from build123d import *

# Parameters (mm, degrees)
SKETCH1_R           = 15.875
SKETCH1_R_2         = 6.35
BOSS_EXTRUDE1_DEPTH = 215.9
BOSS_EXTRUDE2_START = 12.7
SKETCH2_R           = 15.875
SKETCH2_R_2         = 12.7
BOSS_EXTRUDE2_DEPTH = 12.7
SKETCH3_W           = 3.81
SKETCH3_H           = 6.35
CUT_EXTRUDE1_START  = -25.4
SKETCH4_R           = 15.875
CUT_EXTRUDE1_DEPTH  = 25.4


with BuildPart() as part:
    # Sketch1 → Boss-Extrude1 (new body)
    with BuildSketch(Plane(origin=(0, 0, 0), x_dir=(1, 0, 0), z_dir=(0, 1, 0))):
        with Locations(Location((0, 0, 0), (0, 0, 270))):
            Circle(SKETCH1_R)
        with Locations(Location((0, 0, 0), (0, 0, 270))):
            Circle(SKETCH1_R_2, mode=Mode.SUBTRACT)
    extrude(amount=BOSS_EXTRUDE1_DEPTH)

    # Sketch2 → Boss-Extrude2 (add)
    with BuildSketch(Plane.XZ.offset(BOSS_EXTRUDE2_START)):
        with Locations(Location((0, 0, 0), (0, 0, 270))):
            Circle(SKETCH2_R)
        with Locations(Location((0, 0, 0), (0, 0, 270))):
            Circle(SKETCH2_R_2, mode=Mode.SUBTRACT)
    extrude(amount=-BOSS_EXTRUDE2_DEPTH)

    # Sketch3 → Cut-Revolve1 (revolve, cut)
    with BuildSketch(Plane(origin=(0, 0, 0), x_dir=(0, 0, -1), z_dir=(1, 0, 0))):
        with Locations((13.97, 174.625)):
            Rectangle(SKETCH3_W, SKETCH3_H)
    revolve(axis=Axis((0, -12.7, 0), (0, 1, 0)), mode=Mode.SUBTRACT)

    # Sketch4 → Cut-Extrude1 (cut)
    with BuildSketch(Plane(origin=(0, 215.9, 0), x_dir=(1, 0, 0), z_dir=(0, 1, 0)).offset(CUT_EXTRUDE1_START)):
        with Locations(Location((0, 0, 0), (0, 0, 90))):
            Circle(SKETCH4_R)
        Polygon((9.592403624, 11.092300304), (-4.810012038, 13.853415374), (-14.402415662, 2.76111507), (-9.592403624, -11.092300304), (4.810012038, -13.853415374), (14.402415662, -2.76111507), align=None, mode=Mode.SUBTRACT)
    extrude(amount=CUT_EXTRUDE1_DEPTH, mode=Mode.SUBTRACT)


solid = part.part
The listing builds one solid part. Answer for the finished solid, in the listing's coordinates (mm). A direction names the side the tool comes from. Give positions to 0.01 mm unless a question says otherwise; leave off trailing zeros. Order: outer loops, then holes, each group sorted by start corner. A loop starts at its lowest first (then second) coordinate and runs counter-clockwise, first axis right, second up. Notation, with made-up numbers: (-39, 69) - (4, 69) arc R27 ccw to (4, 85) - close; hole circle Ø6 at (-38, 83). An arc over 180 degrees is marked (long way). One line per item, written item: value. Start each with the question number.
1) A cutting plane is placed at C-C on y = 38.5. Give the vertices of the cut face in (x, z) (3 decimals), then the cut area to 3 significant figures.
2) A cutting plane is placed at B-B on x = 0. Give the vertices of the cut face in (y, z) (3 decimals), then the cut area to 3 significant figures.
3) Find the intervals of material crossed by L1, parallel to Y at x = -13.5, z = -7; L2, parallel to X at y = 168, z = 0 (3 decimals); L3, parallel to X at y = -8.5, z = 0 (3 decimals), in increasing order.
4) Given pin 1 Ø3 at (y, z) = (62, 7) entering from +X; pin 2 Ø1 at (x, z) = (-4.5, 9) entering from -Y; pin 3 Ø3 at (y, z) = (123, -6.5) entering from +X, each flat-ended and moving along its own axis, determine where each tip first touches the part or whether it passes through.
5) A tool of negligible diameter and unlimited length cuts with its end or side. For faces 1 (the face through (9.539, 203.022, 8.385)), 2 (the face through (-7.7, -6.4, 10.1)), 3 (the face through (-9.539, 203.022, -8.385)), 4 (the face through (-2.492, 203.022, 12.454)), 5 (the face through (12.03, 203.02, -4.07)), from which of +Z, -Z, +X, -X, +Y, -Y can it reach the whole face along a straight path? Write none if from no direction.
6) The mould has two halves that part along Y. Classify faces 6 (the face through (-12.03, 203.02, 4.07)), 7 (the face through (13, 190.5, -2)), 8 (the face through (-6, 177.8, 11)), 9 (the face through (-6, 171.45, 11)): released by +Y, released by -Y, zero draft, split by the parting line, or undercut.
7) A cutting plane is placed at D-D on z = 8.5. Give the vertices of the cut face in (x, y), then the cut area to 3 significant figures.
8) A cutting plane is placed at A-A on z = 0. Give the vertices of the cut face in (x, y) (3 decimals).
Answer sheet:
1. outline: circle Ø31.75 at (0, 0); hole circle Ø12.7 at (0, 0)
1. area: 665 mm2
2. outline: (-12.7, -15.875) - (171.45, -15.875) - (171.45, -12.065) - (177.8, -12.065) - (177.8, -15.875) - (190.5, -15.875) - (190.5, -12.931) - (215.9, -12.931) - (215.9, -6.35) - (0, -6.35) - (0, -12.7) - (-12.7, -12.7) - close; (-12.7, 12.7) - (0, 12.7) - (0, 6.35) - (215.9, 6.35) - (215.9, 12.931) - (190.5, 12.931) - (190.5, 15.875) - (177.8, 15.875) - (177.8, 12.065) - (171.45, 12.065) - (171.45, 15.875) - (-12.7, 15.875) - close
2. area: 4,000 mm2
3. L1: y = -12.7 to 171.45, 177.8 to 190.5
3. L2: x = -15.875 to -6.35, 6.35 to 15.875
3. L3: x = -15.875 to -12.7, 12.7 to 15.875
4. pin 1: stops at x = 14.89
4. pin 2: stops at y = 0
4. pin 3: stops at x = 15.07
5. face 1: +Z, +X, +Y
5. face 2: -Y
5. face 3: -Z, -X, +Y
5. face 4: +Z, -X, +Y
5. face 5: -Z, +X, +Y
6. face 6: zero draft
6. face 7: released by +Y
6. face 8: undercut
6. face 9: undercut
7. outline: (-13.41, -12.7) - (-9.44, -12.7) - (-9.44, 0) - (9.44, 0) - (9.44, -12.7) - (13.41, -12.7) - (13.41, 171.45) - (8.56, 171.45) - (8.56, 177.8) - (13.41, 177.8) - (13.41, 190.5) - (9.44, 190.5) - (9.44, 215.9) - (-10.49, 215.9) - (-10.49, 190.5) - (-13.41, 190.5) - (-13.41, 177.8) - (-8.56, 177.8) - (-8.56, 171.45) - (-13.41, 171.45) - close
7. area: 5,650 mm2
8. outline: (-15.875, -12.7) - (-12.7, -12.7) - (-12.7, 0) - (-6.35, 0) - (-6.35, 215.9) - (-13.444, 215.9) - (-13.444, 190.5) - (-15.875, 190.5) - (-15.875, 177.8) - (-12.065, 177.8) - (-12.065, 171.45) - (-15.875, 171.45) - close; (6.35, 0) - (12.7, 0) - (12.7, -12.7) - (15.875, -12.7) - (15.875, 171.45) - (12.065, 171.45) - (12.065, 177.8) - (15.875, 177.8) - (15.875, 190.5) - (13.444, 190.5) - (13.444, 215.9) - (6.35, 215.9) - close
